Could you check a few things on this model? Use its own coordinates, in mm. A direction names the side the tool comes from. Round coordinates to 2 decimals unless told otherwise and drop trailing zeros. Write each loop counter-clockwise with the first axis right and the second up, starting at its lowest first coordinate (ties: lowest second). Pieces come first, ordered by that corner, then holes. Notation, with made-up numbers: (9.5, 15.25) - (40.5, 15.25) arc R22 ccw to (40.5, 28.25) - close; hole circle Ø8 at (3.5, -12). An arc over 180 degrees is marked (long way). Write each question's results on one line, items separated by ' | '. Start each with the question number.
(1) For P1, Ø4.5, axis at x = -17, z = 18, coming from the +Y side; P2, Ø2, axis at y = 2, z = -43.5, coming from the +X side; P3, Ø1, axis at x = -9.5, z = 26.5, coming from the +Y side; P4, Ø3, axis at x = -35, z = -34, coming from the -Y side, each with a flat end and sliding along its axis, tell me the tip position at first contact or that it passes through.
(2) Thinking about a two-plate mould opening in Z: for faces 4 (the cylindrical face through (-43, 5, -39)), 5 (the flat face through (-5.04, 1.53, -80.56)), 6 (the cylindrical face through (43, 5, 39)), which applies, +Z half, -Z half, draft (parallel to the pull), parting line (faces both ways), or undercut?
(3) Please list where these lines run through material, in increasing order: line 1 (X direction, y = 9.4, z = 34); line 2 (Z direction, x = 0, y = 7.55); line 3 (X direction, y = 3, z = 19). Write a range as [from, to].
(4) Imagine slicing it at C-C on z = 19. Write out the boundary of the cut face in (x, y), then the cut area to 3 significant figures.
(5) Imagine slicing it at B-B on x = -35. Write out the boundary of the cut face in (y, z).
(6) On a 3-axis mill with a long thin cutter (end or side, diameter ignored), from which of +Z, -Z, +X, -X, +Y, -Y can I reach the whole of each face in a straight line? I mean faces 1 (the cylindrical face through (-15.5, 3.5, -68.8)), 2 (the flat face through (4, 5, -4)), 3 (the flat face through (7, 8.6, 14)). Say none if no direction works.
Autodesk Inventor part; units mm, degrees
ref_plane "YZ Plane" through (0, 0, 0) normal (1, 0, 0) x (0, 1, 0)
ref_plane "XZ Plane" through (0, 0, 0) normal (0, 1, 0) x (-1, 0, 0)
ref_plane "XY Plane" through (0, 0, 0) normal (0, 0, 1) x (1, 0, 0)
sketch "Boceto1" plane through (0, 0, 0) normal (0, 1, 0) x (-1, 0, 0)
  circle A0 centre (0, 0) radius 4.35
  line L0 (-45, 40) -> (45, 40)
  line L1 (45, 40) -> (45, -40)
  line L2 (45, -40) -> (-45, -40)
  line L3 (-45, -40) -> (-45, 40)
  line L4 (-45, 40) -> (45, -40) construction
  line L5 (45, 40) -> (-45, -40) construction
  dimension "d0" = 8.7
  dimension "d1" = 80
  dimension "d2" = 90
extrude "Extrusión1" add sketch "Boceto1" along normal blind 10
sketch "Boceto2" plane through (0, 10, 0) normal (0, 1, 0) x (1, 0, 0)
  circle A0 centre (0, 0) radius 4.35
  circle A1 centre (0, 0) radius 32.875
  dimension "d5" = 65.75
extrude "Extrusión2" cut sketch "Boceto2" against normal blind 1.4
sketch "Boceto3" plane through (0, 8.6, 0) normal (0, 1, 0) x (1, 0, 0)
  circle A0 centre (0, 0) radius 4.35
  circle A1 centre (0, 0) radius 15
  dimension "d8" = 30
extrude "Extrusión3" add sketch "Boceto3" along normal up to surface (1.4 mm away)
sketch "Boceto4" plane through (0, 8.6, 0) normal (0, 1, 0) x (1, 0, 0)
  circle A0 centre (0, -18.25) radius 2.65
  circle A1 centre (0, 18.25) radius 2.65
  point P0 (0, 0)
  dimension "d11" = 5.3
  dimension "d12" = 36.5
  dimension "d13" = 18.25
extrude "Extrusión4" [suppressed]
sketch "Boceto5" plane through (0, 8.6, 0) normal (0, 1, 0) x (1, 0, 0)
  circle A0 centre (0, -18.25) radius 2.65
  circle A1 centre (0, -18.25) radius 4.05
  circle A2 centre (0, 18.25) radius 2.65
  circle A3 centre (0, 18.25) radius 4.05
  line L0 (-4.6765, -18.25) -> (-2.3383, -14.2)
  line L1 (-2.3383, -14.2) -> (2.3383, -14.2)
  line L2 (2.3383, -14.2) -> (4.6765, -18.25)
  line L3 (4.6765, -18.25) -> (2.3383, -22.3)
  line L4 (2.3383, -22.3) -> (-2.3383, -22.3)
  line L5 (-2.3383, -22.3) -> (-4.6765, -18.25)
  line L6 (-4.6765, 18.25) -> (-2.3383, 22.3)
  line L7 (-2.3383, 22.3) -> (2.3383, 22.3)
  line L8 (2.3383, 22.3) -> (4.6765, 18.25)
  line L9 (4.6765, 18.25) -> (2.3383, 14.2)
  line L10 (2.3383, 14.2) -> (-2.3383, 14.2)
  line L11 (-2.3383, 14.2) -> (-4.6765, 18.25)
  point P0 (0, 0)
  dimension "d16" = 8.1
extrude "Extrusión5" [suppressed]
sketch "Boceto6" plane through (0, 10, 0) normal (0, 1, 0) x (1, 0, 0)
  circle A0 centre (-35, 34) radius 2.7
  circle A1 centre (35, 34) radius 2.7
  circle A2 centre (-35, -34) radius 2.7
  circle A3 centre (35, -34) radius 2.7
  line L0 (-45, 40) -> (-45, -40)
  line L1 (45, 40) -> (-45, 40)
  line L2 (-45, -40) -> (45, -40)
  line L3 (45, -40) -> (45, 40)
  point P0 (0, 0)
  dimension "d19" = 5.4
  dimension "d20" = 10
  dimension "d21" = 6
  dimension "d22" = 6
  dimension "d23" = 10
extrude "Extrusión6" cut sketch "Boceto6" against normal through all contours A0 | A1 | A2 | A3
fillet "Empalme1" radius 5 4 edges at (45, 5, 40) (45, 5, -40) (-45, 5, 40) (-45, 5, -40)
sketch "Boceto7" plane through (0, 10, 0) normal (0, 1, 0) x (1, 0, 0)
  circle A0 centre (-35, -34) radius 2.7
  circle A1 centre (-35, -34) radius 4.7
  circle A2 centre (35, -34) radius 2.7
  circle A3 centre (35, -34) radius 4.7
  circle A4 centre (35, 34) radius 2.7
  circle A5 centre (35, 34) radius 4.7
  circle A6 centre (-35, 34) radius 2.7
  circle A7 centre (-35, 34) radius 4.7
  point P0 (0, 0)
  dimension "d27" = 9.4
extrude "Extrusión7" cut sketch "Boceto7" against normal blind 2.1 contours A0 | A1 | A2 | A3 | A4 | A5 | A6 | A7
sketch "Boceto9" plane through (0, 0, 0) normal (0, -1, 0) x (1, 0, 0)
  circle A0 centre (0, 0) radius 4.35
  circle A1 centre (0, 0) radius 8.175
  dimension "d32" = 16.35
extrude "Extrusión9" cut sketch "Boceto9" against normal blind 5 contours A0 | A1
sketch "Boceto10" plane through (0, 8.6, 0) normal (0, 1, 0) x (1, 0, 0)
  circle A0 centre (19, -19) radius 2.7
  line L0 (26, 26) -> (-26, 26)
  line L1 (-26, 26) -> (-26, -26)
  line L2 (-26, -26) -> (26, -26)
  line L3 (26, -26) -> (26, 26)
  circle A1 centre (0, 0) radius 4.35
  line L4 (26, 26) -> (-26, -26) construction
  line L5 (-26, 26) -> (26, -26) construction
  circle A2 centre (0, 0) radius 15
  circle A3 centre (0, 0) radius 21
  circle A4 centre (19, -19) radius 5
  line L6 (-19, 19) -> (19, 19)
  line L7 (19, 19) -> (19, -19)
  line L8 (19, -19) -> (-19, -19)
  line L9 (-19, -19) -> (-19, 19)
  line L10 (-19, 19) -> (19, -19) construction
  line L11 (19, 19) -> (-19, -19) construction
  dimension "d35" = 52
  dimension "d36" = 52
  dimension "d37" = 42
  dimension "d38" = 5.4
  dimension "d39" = 10
  dimension "d40" = 38
extrude "Extrusión10" cut sketch "Boceto10" against normal through all contours A0 L8 L7 | L7 L8 A0
sketch "Boceto11" plane through (0, 8.6, 0) normal (0, 1, 0) x (1, 0, 0)
  circle A0 centre (19, -19) radius 2.7
  circle A1 centre (19, -19) radius 4.7
  point P0 (0, 0)
  dimension "d43" = 9.4
extrude "Extrusión11" cut sketch "Boceto11" against normal blind 2.3
pattern_circular "Patrón circular1" count 4 over 360 about axis through (0, 8.6, 0) along (0, 1, 0) of "Extrusión10", "Extrusión11"
sketch "Boceto12" plane through (0, 10, 0) normal (0, 1, 0) x (1, 0, 0)
  line L0 (40, 40) -> (-40, 40)
  line L1 (25, 40) -> (-25, 40)
  line L2 (-25, 40) -> (-25, 87)
  line L3 (-25, 87) -> (25, 87)
  line L4 (25, 87) -> (25, 40)
  point P0 (0, 0)
  point P1 (-25, 40)
  dimension "d49" = 25
  dimension "d50" = 25
  dimension "d51" = 47
extrude "Extrusión12" add sketch "Boceto12" against normal up to surface (10 mm away)
fillet "Empalme2" radius 5 4 edges at (25, 5, -40) (25, 5, -87) (-25, 5, -87) (-25, 5, -40)
sketch "Boceto13" plane through (0, 10, 0) normal (0, 1, 0) x (1, 0, 0)
  circle A0 centre (0, 55) radius 8.5
  circle A1 centre (0, 65) radius 8.5
  line L0 (-8.5, 55) -> (8.5, 55)
  line L1 (8.5, 55) -> (8.5, 65)
  line L2 (8.5, 65) -> (-8.5, 65)
  line L3 (-8.5, 65) -> (-8.5, 55)
  line L4 (20, 87) -> (-20, 87)
  point P0 (0, 0)
  point P1 (-8.5, 65)
  dimension "d55" = 17
  dimension "d57" = 10
  dimension "d93" = 55
extrude "Extrusión13" cut sketch "Boceto13" against normal through all
sketch "Boceto14" plane through (0, 10, 0) normal (0, 1, 0) x (1, 0, 0)
  circle A0 centre (-15.5, 39.5) radius 1.7
  line L0 (-17.2, 39.5) -> (-13.8, 39.5)
  line L1 (-13.8, 39.5) -> (-13.8, 49.5)
  line L2 (-13.8, 49.5) -> (-17.2, 49.5)
  line L3 (-17.2, 49.5) -> (-17.2, 39.5)
  circle A1 centre (-15.5, 49.5) radius 1.7
  arc A2 (-8.5, 55) -> (8.5, 55) centre (0, 55) ccw
  line L4 (0, 55) -> (-15.5, 55)
  line L5 (-15.5, 55) -> (-15.5, 39.5)
  line L6 (-15.5, 39.5) -> (0, 39.5)
  line L7 (0, 39.5) -> (0, 55)
  point P0 (0, 0)
  dimension "d62" = 3.4
  dimension "d60" = 15.5
  dimension "d61" = 15.5
  dimension "d63" = 10
extrude "Extrusión14" cut sketch "Boceto14" against normal through all contours L0 A0 | L3 A1 L5 A0 | A0 L5 L0 | L0 L5 A0 | A0 L5 A1 L1 | A1 L5 L2 | L2 L5 A1 | A1 L5 L2 | L2 L5 A1
pattern_linear "Patrón rectangular1" count 2 spacing 31 along (0, 0, -1) count 2 spacing 31 along (1, 0, 0) of "Extrusión14"
sketch "Boceto15" plane through (0, 10, 0) normal (0, 1, 0) x (1, 0, 0)
  arc A0 (-17.2, 39.5) -> (-13.8, 39.5) centre (-15.5, 39.5) ccw
  line L0 (-17.2, 39.5) -> (-17.2, 49.5)
  line L1 (-13.8, 49.5) -> (-13.8, 39.5)
  arc A1 (-13.8, 49.5) -> (-17.2, 49.5) centre (-15.5, 49.5) ccw
  line L2 (-18.7, 49.5) -> (-18.7, 39.5)
  arc A2 (-18.7, 39.5) -> (-12.3, 39.5) centre (-15.5, 39.5) ccw
  line L3 (-12.3, 39.5) -> (-12.3, 49.5)
  arc A3 (-12.3, 49.5) -> (-18.7, 49.5) centre (-15.5, 49.5) ccw
  point P0 (0, 0)
  point P1 (-17.2, 28.0165)
  point P2 (-13.8, 29.8383)
  dimension "d72" = 1.5
extrude "Extrusión15" cut sketch "Boceto15" against normal blind 3 contours L0 A1 L1 A0 | A3 L3 A2 L2
pattern_linear "Patrón rectangular2" count 2 spacing 31 along (0, 0, -1) count 2 spacing 31 along (1, 0, 0) of "Extrusión15"
sketch "Boceto16" plane through (0, 10, 0) normal (0, 1, 0) x (1, 0, 0)
  circle A0 centre (-7.5, 82) radius 1.7
  circle A1 centre (7.5, 82) radius 1.7
  arc A2 (8.5, 65) -> (-8.5, 65) centre (0, 65) ccw
  line L0 (20, 87) -> (-20, 87)
  point P0 (0, 0)
  dimension "d81" = 3.4
  dimension "d82" = 15
  dimension "d83" = 7.5
  dimension "d84" = 5
extrude "Extrusión16" cut sketch "Boceto16" against normal through all
sketch "Boceto17" plane through (0, 0, 0) normal (0, -1, 0) x (1, 0, 0)
  circle A0 centre (-7.5, -82) radius 1.7
  circle A1 centre (-7.5, -82) radius 2.85
  circle A2 centre (7.5, -82) radius 1.7
  circle A3 centre (7.5, -82) radius 2.85
  line L0 (-4.2091, -82) -> (-5.8546, -84.85)
  line L1 (-5.8546, -84.85) -> (-9.1454, -84.85)
  line L2 (-9.1454, -84.85) -> (-10.7909, -82)
  line L3 (-10.7909, -82) -> (-9.1454, -79.15)
  line L4 (-9.1454, -79.15) -> (-5.8546, -79.15)
  line L5 (-5.8546, -79.15) -> (-4.2091, -82)
  line L6 (10.7909, -82) -> (9.1454, -84.85)
  line L7 (9.1454, -84.85) -> (5.8546, -84.85)
  line L8 (5.8546, -84.85) -> (4.2091, -82)
  line L9 (4.2091, -82) -> (5.8546, -79.15)
  line L10 (5.8546, -79.15) -> (9.1454, -79.15)
  line L11 (9.1454, -79.15) -> (10.7909, -82)
  point P0 (0, 0)
  dimension "d87" = 5.7
extrude "Extrusión17" cut sketch "Boceto17" against normal blind 3.1 contours A0 | A1 | A1 L5 L0 | A1 L4 L5 | L0 L1 A1 | A1 L3 L4 | L1 L2 A1 | A1 L2 L3 | A2 | A3 | A3 L11 L6 | A3 L10 L11 | L6 L7 A3 | A3 L9 L10 | L7 L8 A3 | A3 L8 L9
sketch "Boceto8" plane through (0, 10, 0) normal (0, 1, 0) x (1, 0, 0)
  line L0 (4.981, 25.0262) -> (-4.981, 25.0262)
  line L1 (-4.981, 25.0262) -> (-4.981, 54.9738)
  line L2 (-4.981, 54.9738) -> (4.981, 54.9738)
  line L3 (4.981, 54.9738) -> (4.981, 25.0262)
  line L4 (40, 40) -> (-40, 40)
  line L5 (4.981, 25.0262) -> (-4.981, 54.9738) construction
  line L6 (-4.981, 25.0262) -> (4.981, 54.9738) construction
  point P0 (0, 0)
  point P1 (0, 40)
properties part number "Shoulderbasetop"
Response:
1) P1: y = 6.3 | P2: x = 25.67 | P3: y = 8.6 | P4: through
2) face 4: -Z half | face 5: undercut | face 6: +Z half
3) line 1: [-45, -39.7], [-30.3, 30.3], [39.7, 45] | line 2: [-87, -73.5], [-46.5, -4.35], [4.35, 40] | line 3: [-45, -21.7], [-16.3, 16.3], [21.7, 45]
4) outline: (-45, 0) - (-21.7, 0) - (-21.7, 6.3) - (-23.7, 6.3) - (-23.7, 8.6) - (-26.83, 8.6) - (-26.83, 10) - (-45, 10) - close; (-16.3, 0) - (16.3, 0) - (16.3, 6.3) - (14.3, 6.3) - (14.3, 8.6) - (-14.3, 8.6) - (-14.3, 6.3) - (-16.3, 6.3) - close; (21.7, 0) - (45, 0) - (45, 10) - (26.83, 10) - (26.83, 8.6) - (23.7, 8.6) - (23.7, 6.3) - (21.7, 6.3) - close | area: 714 mm²
5) outline: (0, -40) - (10, -40) - (10, -38.7) - (7.9, -38.7) - (7.9, -36.7) - (0, -36.7) - close; (0, -31.3) - (7.9, -31.3) - (7.9, -29.3) - (10, -29.3) - (10, 29.3) - (7.9, 29.3) - (7.9, 31.3) - (0, 31.3) - close; (0, 36.7) - (7.9, 36.7) - (7.9, 38.7) - (10, 38.7) - (10, 40) - (0, 40) - close
6) face 1: +Y, -Y | face 2: -Y | face 3: +Y
